from build123d import *

# Parameters (mm, degrees)
BOSS_EXTRUDE1_DEPTH = 300
SKETCH2_R           = 2
CUT_EXTRUDE1_DEPTH  = 5
FILLET1_R           = 1
FILLET2_R           = 1


with BuildPart() as part:
    # Sketch1 → Boss-Extrude1 (new body)
    with BuildSketch(Plane.XY):
        Polygon((-11, 5), (-11, 0), (11, 0), (11, 5), (20.5, 5), (20.5, -5), (-20.5, -5), (-20.5, 5), align=None)
    extrude(amount=BOSS_EXTRUDE1_DEPTH)

    # Sketch2 → Cut-Extrude1 (cut)
    with BuildSketch(Plane.XZ.offset(5)):
        with Locations((-14.5, 293)):
            Circle(SKETCH2_R)
        with Locations((0, 293)):
            Circle(SKETCH2_R)
        with Locations((14.5, 293)):
            Circle(SKETCH2_R)
        with Locations((0, 266)):
            Circle(SKETCH2_R)
        with Locations((0, 250)):
            Circle(SKETCH2_R)
        with Locations((0, 233)):
            Circle(SKETCH2_R)
        with Locations((0, 169)):
            Circle(SKETCH2_R)
        with Locations((0, 105)):
            Circle(SKETCH2_R)
        with Locations((0, 186)):
            Circle(SKETCH2_R)
        with Locations((0, 122)):
            Circle(SKETCH2_R)
        with Locations((0, 202)):
            Circle(SKETCH2_R)
        with Locations((0, 138)):
            Circle(SKETCH2_R)
        with Locations((0, 74)):
            Circle(SKETCH2_R)
        with Locations((0, 58)):
            Circle(SKETCH2_R)
        with Locations((0, 41)):
            Circle(SKETCH2_R)
    extrude(amount=-CUT_EXTRUDE1_DEPTH, mode=Mode.SUBTRACT)

    # Fillet1
    fillet1_edges = [part.edges().sort_by_distance(p)[0] for p in [
        (20.5, 5, 150),
        (20.5, -5, 150),
        (-20.5, -5, 150),
        (-20.5, 5, 150),
        (-11, 5, 150),
        (11, 5, 150),
    ]]
    fillet(fillet1_edges, radius=FILLET1_R)

    # Fillet2
    fillet2_edges = [part.edges().sort_by_distance(p)[0] for p in [
        (0, 0, 300),
        (20.207106781, -4.707106781, 300),
        (-11.292893219, 4.707106781, 300),
        (11.292893219, 4.707106781, 300),
        (-11, 2, 300),
        (11, 2, 0),
        (11, 2, 300),
        (15.75, 5, 0),
        (20.5, 0, 0),
        (0, -5, 0),
        (-20.5, 0, 0),
        (-15.75, 5, 0),
        (20.207106781, 4.707106781, 0),
        (-20.207106781, 4.707106781, 0),
        (-20.207106781, -4.707106781, 0),
        (20.207106781, -4.707106781, 0),
        (-11, 2, 0),
        (-11.292893219, 4.707106781, 0),
        (11.292893219, 4.707106781, 0),
        (15.75, 5, 300),
        (-15.75, 5, 300),
        (-20.5, 0, 300),
        (0, 0, 0),
        (0, -5, 300),
        (20.5, 0, 300),
        (20.207106781, 4.707106781, 300),
        (-20.207106781, 4.707106781, 300),
        (-20.207106781, -4.707106781, 300),
    ]]
    fillet(fillet2_edges, radius=FILLET2_R)


solid = part.part
For this review, take the finished solid that the model builds, in its own axes (mm). A direction names the side the tool comes from. Coordinates: 2 decimals unless noted, no trailing zeros. Loops run counter-clockwise (first coordinate to the right, second up) from the corner with the lowest first, then second, coordinate; pieces in that order, holes last. Notation, with made-up numbers: (-32.5, -26) - (13.5, -26) arc R25 cw to (13.5, 7) - close; hole circle Ø11 at (-5.5, 25.25). An arc over 180 degrees is marked (long way). Use a Markdown table: item, result. Add a question column.
Item 1: Insertion check: pin 1 Ø11 at (x, z) = (5, 89) entering from +Y. The pin has a flat end and moves straight along its axis. Give the tip position at first contact, or say it passes through.
Item 2: Tool access review of faces 1 (the face through (0, 0, 148)), 2 (the face through (-20.5, 0, 148)): name each direction out of +Z, -Z, +X, -X, +Y, -Y from which nothing blocks a thin tool from reaching the whole face with its end or side.
Item 3: We need section A-A (x = -8.5). Give the boundary of the cut face in (y, z).
Item 4: We need section B-B (z = 81.5). Give the boundary of the cut face in (x, y), and give its area (3 significant figures).
Item 5: For line 1 (X direction, y = -1.3, z = 293); line 2 (X direction, y = 2.25, z = 18.5); line 3 (Z direction, x = -14.5, y = -1.6), list the stretches that pass through material, from the lowest coordinate up.
Results list:
| question | item | result |
|---|---|---|
| 1 | pin 1 | stops at y = 0 |
| 2 | face 1 | +Z, -Z, +Y |
| 2 | face 2 | +Z, -Z, -X, +Y, -Y |
| 3 | outline | (-5, 1) arc R1 ccw to (-4, 0) - (-1, 0) arc R1 ccw to (0, 1) - (0, 299) arc R1 ccw to (-1, 300) - (-4, 300) arc R1 ccw to (-5, 299) - close |
| 4 | outline | (-20.5, -4) arc R1 ccw to (-19.5, -5) - (19.5, -5) arc R1 ccw to (20.5, -4) - (20.5, 4) arc R1 ccw to (19.5, 5) - (12, 5) arc R1 ccw to (11, 4) - (11, 0) - (-11, 0) - (-11, 4) arc R1 ccw to (-12, 5) - (-19.5, 5) arc R1 ccw to (-20.5, 4) - close |
| 4 | area | 299 mm^2 |
| 5 | line 1 | x = -20.5 to -16.5, -12.5 to -2, 2 to 12.5, 16.5 to 20.5 |
| 5 | line 2 | x = -20.5 to -11, 11 to 20.5 |
| 5 | line 3 | z = 0 to 291, 295 to 300 |
